Source: CAD feature listing. Evaluate the final solid. Frame: model axes, mm. Face numbers are marked on the shaded views. A direction names the side the tool comes from. Give positions to 0.01 mm unless a question says otherwise; leave off trailing zeros. Loops run counter-clockwise (first coordinate to the right, second up) from the corner with the lowest first, then second, coordinate; pieces in that order, holes last.
Autodesk Inventor part; units mm, degrees
ref_plane "YZ Plane" through (0, 0, 0) normal (1, 0, 0) x (0, 1, 0)
ref_plane "XZ Plane" through (0, 0, 0) normal (0, 1, 0) x (-1, 0, 0)
ref_plane "XY Plane" through (0, 0, 0) normal (0, 0, 1) x (1, 0, 0)
sketch "Skizze1" plane through (0, 0, 0) normal (0, 0, 1) x (1, 0, 0)
  line L0 (0, 0) -> (0, 22)
  line L1 (0, 22) -> (5, 22)
  line L2 (5, 22) -> (5, 5)
  line L3 (5, 5) -> (23.5, 5)
  line L4 (23.5, 5) -> (23.5, 22)
  line L5 (23.5, 22) -> (28.5, 22)
  line L6 (28.5, 22) -> (28.5, 0)
  line L7 (28.5, 0) -> (0, 0)
  line L8 (14.25, 5) -> (14.25, 0) construction
  line L9 (0, 11.55) -> (28.5, 11.55) construction
  dimension "d0" = 5
  dimension "d1" = 5
  dimension "d2" = 11.55
  dimension "d3" = 18.5
  dimension "d4" = 22
  dimension "d14" = 28.5
extrude "Extrusion1" add sketch "Skizze1" along normal blind 25
sketch "Skizze2" plane through (28.5, 0, 0) normal (1, 0, 0) x (0, 0, -1)
  circle A0 centre (-12.5, 11.25) radius 5
  line L0 (-12.5, 11.25) -> (-12.5, 22) construction
  line L1 (0, 22) -> (-25, 22) construction
  circle A1 centre (-12.5, 11.25) radius 6.5
  point P0 (0, 0)
  point P1 (-25, 0)
  dimension "d7" = 11.25
  dimension "d8" = 10
  dimension "d20" = 13
extrude "Extrusion2" cut sketch "Skizze2" against normal through all contours A0
sketch "Skizze3" plane through (5, 5, 0) normal (0, 1, 0) x (1, 0, 0)
  line L0 (18.5, -25) -> (0, -25) construction
  line L1 (9.25, -25) -> (9.25, 0) construction
  line L2 (18.5, 0) -> (0, 0) construction
  line L3 (9.25, -44.3) -> (9.25, -5.7) construction
  line L4 (18.5, -44.3) -> (18.5, -5.7)
  line L5 (0, -5.7) -> (0, -44.3)
  arc A0 (0, -44.3) -> (18.5, -44.3) centre (9.25, -44.3) ccw
  arc A1 (18.5, -5.7) -> (0, -5.7) centre (9.25, -5.7) ccw
  line L6 (29.2, -12.5) -> (-10.7, -12.5) construction
  line L7 (8, 0) -> (8, -25) construction
  line L8 (18, 0) -> (18, -25) construction
  line L9 (0, -25) -> (-5, -25)
  line L10 (9.25, 0) -> (1.9649, 0)
  line L11 (18.5, 0) -> (0, 0)
  line L12 (-5, 0) -> (23.5, 0)
  line L13 (18.5, 0) -> (18.5, -5.7)
  line L14 (0, 0) -> (0, -5.7)
  point P0 (16.5351, 0)
  dimension "d11" = 18.5
  dimension "d25" = 6.8
  dimension "d32" = 0.5
  dimension "d33" = 10
extrude "Extrusion3" cut sketch "Skizze3" against normal through all
sketch "Skizze4" plane through (5, 5, 0) normal (0, 1, 0) x (1, 0, 0)
  line L0 (18.5, 0) -> (0, 0)
  line L1 (9.25, -11) -> (9.25, 19) construction
  line L2 (-5, 0) -> (23.5, 0)
  line L3 (0, -11) -> (0, 19)
  line L4 (18.5, 19) -> (18.5, -11)
  arc A0 (0, -11) -> (18.5, -11) centre (9.25, -11) ccw
  arc A1 (18.5, 19) -> (0, 19) centre (9.25, 19) ccw
  line L5 (6.5, 19) -> (6.5, -11)
  arc A2 (6.5, -11) -> (12, -11) centre (9.25, -11) ccw
  line L6 (12, -11) -> (12, 19)
  arc A3 (12, 19) -> (6.5, 19) centre (9.25, 19) ccw
  arc A4 (6.5, 6.75) -> (12, 6.75) centre (9.25, 6.75) ccw
  line L7 (23.5, -11) -> (23.5, 19)
  arc A5 (23.5, 19) -> (-5, 19) centre (9.25, 19) ccw
  line L8 (-5, 19) -> (-5, -11)
  arc A6 (-5, -11) -> (23.5, -11) centre (9.25, -11) ccw
  arc A7 (18.5, 0) -> (0, 0) centre (9.25, -11.8084) ccw
  point P0 (9.25, 4)
  point P1 (18.5, 0)
  point P2 (6.5, 0)
  point P3 (12, 0)
  point P4 (8.25, 0)
  point P5 (9.25, 0)
  point P6 (18.5, -5.7)
  point P7 (0, -5.7)
  point P8 (0, -5.7)
  dimension "d15" = 15
  dimension "d18" = 5.5
  dimension "d26" = 4
  dimension "d34" = 5
  dimension "d35" = 15
extrude "Extrusion4" add sketch "Skizze4" against normal up to surface (5 mm away) contours L4 A1 L3 L2 L8 A5 L7 | A7 L6 A3 L5 L3 A1 L4 | L0 L6 A7 | L0 L5 A7 L6 | A7 L5 A4 L6 | L0 A7 L5
extrude "Extrusion5" cut sketch "Skizze2" against normal blind 5
extrude "Extrusion6" cut sketch "Skizze2" along normal blind 5 from surface at -28.5
chamfer "Fase1" distance 6 angle 45 4 edges at (26, 22, 25) (2.5, 22, 25) (2.5, 22, 0) (26, 22, 0)
fillet "Rundung4" radius 6 2 edges at (26, 5, 0) (2.5, 5, 0)
ref_plane "Arbeitsebene2" through (14.25, 0, -19) normal (1, 0, 0) x (0, 0, -1)
fillet "Rundung5" radius 3 1 edges at (14.25, 5, 0)
properties part number "BeltDiscBottomPart"
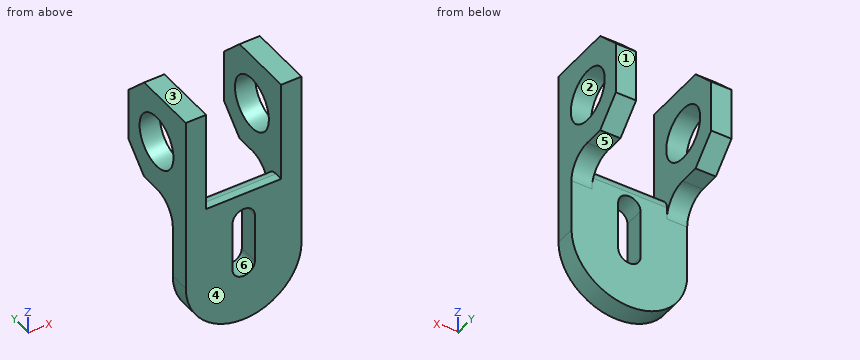
1) Pull-direction query (Z, two-part tool) for the marked faces 1, 2 and 3; classes: released by +Z, released by -Z, zero draft, split by the parting line, or undercut.
Checks:
face 1: zero draft
face 2: undercut
face 3: released by +Z
2) Contact query for flat-ended pins moving along their axis: P1, Ø4, axis at x = 25.5, y = 13.5, coming from the -Z side; P2, Ø3, axis at x = 23, z = -9, coming from the +Y side; P3, Ø2, axis at x = 14.5, y = 0.5, coming from the +Z side; P4, Ø8, axis at x = 10, z = 6, coming from the +Y side. Output: stop coordinate, or through.
Checks:
P1: stops at z = 0
P2: stops at y = 5
P3: stops at z = 0
P4: passes through
3) Cut plane D-D (z = 12.5). Return loops of the section in (x, y), and give its area (3 significant figures).
Checks:
outline: (0, 0) - (5, 0) - (5, 4.75) - (0, 4.75) - close; (0, 17.75) - (5, 17.75) - (5, 22) - (0, 22) - close; (23.5, 0) - (28.5, 0) - (28.5, 4.75) - (23.5, 4.75) - close; (23.5, 17.75) - (28.5, 17.75) - (28.5, 22) - (23.5, 22) - close
area: 90.0 mm2
4) Cut plane B-B (z = -9). Return loops of the section in (x, y).
Checks:
outline: (0, 0) - (11.5, 0) - (11.5, 5) - (0, 5) - close; (17, 0) - (28.5, 0) - (28.5, 5) - (17, 5) - close
5) Ray query, probe 1 along X at (y, z) = (14.5, 22.5); probe 2 along Y at (x, z) = (1.5, 12.5); probe 3 along Z at (x, y) = (3.75, 11). Return the intervals inside material, ascending.
Checks:
probe 1: x = 0 to 5, 23.5 to 28.5
probe 2: y = 0 to 4.75, 17.75 to 22
probe 3: z = 0 to 6, 19 to 25
6) Cut plane C-C (x = 14.25). Return loops of the section in (y, z), and give its area (3 significant figures).
Checks:
outline: (0, -33.25) - (5, -33.25) - (5, -21.75) - (0, -21.75) - close; (0, -4) - (5, -4) - (5, -3) arc R3 ccw to (2, 0) - (0, 0) - close
area: 75.6 mm2
7) Reachability of the marked faces 4, 5 and 6 from +Z, -Z, +X, -X, +Y, -Y: full face, straight path, thin tool, end or side. Return the list, or none.
Checks:
face 4: +Z, -Z, +X, -X, -Y
face 5: -Z, +X, -X, +Y
face 6: +Y, -Y
8) Cut plane A-A (y = 19.75). Return loops of the section in (x, z), and give its area (3 significant figures).
Checks:
outline: (0, 3.75) - (5, 3.75) - (5, 21.25) - (0, 21.25) - close; (23.5, 3.75) - (28.5, 3.75) - (28.5, 21.25) - (23.5, 21.25) - close
area: 175 mm2
